```python
from build123d import *

# Parameters (mm, degrees)
BOX_W     = 13.4
BOX_H     = 13.4
BOX_DEPTH = 14


with BuildPart() as cube:
    # Box → Box (new body)
    with BuildSketch(Plane(origin=(-6.7, -6.7, 10), x_dir=(1, 0, 0), z_dir=(0, 0, 1))):
        with Locations((6.7, 6.7)):
            Rectangle(BOX_W, BOX_H)
    extrude(amount=BOX_DEPTH)


with BuildPart() as cut:
    # Sketch → Revolve (revolve)
    with BuildSketch(Plane.XZ):
        with BuildLine():
            Line((118.075, 18.37), (129.708369, 18.37))
            Line((129.708369, 18.37), (121.740684, 21.27))
            Line((121.740684, 21.27), (121.740684, 23.77))
            Line((121.740684, 23.77), (129.708369, 26.67))
            Line((129.708369, 26.67), (4.86, 26.67))
            Line((4.86, 26.67), (4.86, 10.010664))
            Line((4.86, 10.010664), (11.05, 10.010664))
            Line((11.05, 10.010664), (11.05, 18.37))
            add(Edge.make_bspline(
                [(118.075, 18.37), (77.146439, 24.763197), (51.362286, 25.0243), (11.05, 18.37)],
                knots=[0, 0, 0, 0, 1, 1, 1, 1], degree=3))
        make_face()
    revolve(axis=Axis((0, 0, 0), (0, 0, 1)))

    # Cut: cut Cube
    add(cube.part, mode=Mode.SUBTRACT)


solid = cut.part
```
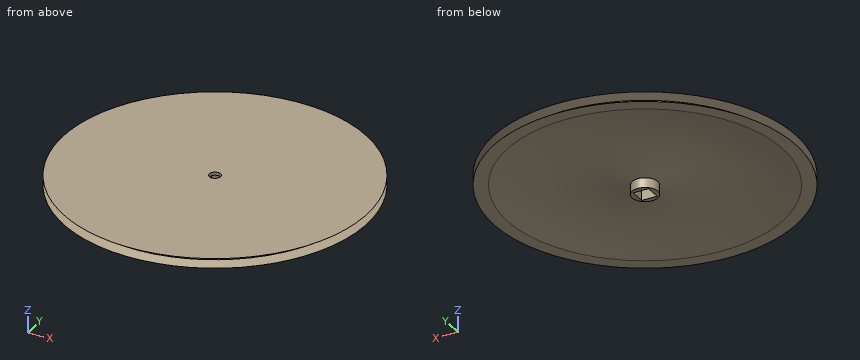
Geometry check sheet. Reference: the model listing, model coordinates, mm. Give positions to 0.01 mm unless a question says otherwise; leave off trailing zeros. Write each loop counter-clockwise with the first axis right and the second up, starting at its lowest first coordinate (ties: lowest second). Pieces come first, ordered by that corner, then holes.
1) Material ranges on L1, parallel to Z at x = -110, y = 29; L2, parallel to Z at x = 54, y = -58, recorded low to high.
2) Section check A-A, the plane z = 15.75. Record the boundary of the cut face in (x, y).
3) Gauge pin test, flat ends, axial feed: pin 1 (1 mm diameter, centred on x = -9, z = 15.5, fed in from +Y); pin 2 (4 mm diameter, centred on y = -1, z = 13.5, fed in from -X); pin 3 (10 mm diameter, centred on x = 10.5, y = -37.5, fed in from -Z). Record the tip position at first contact, or that the pin passes through.
Computed:
1. L1: z = 19.03 to 26.67
1. L2: z = 22.8 to 26.67
2. outline: circle Ø22.1 at (0, 0); hole (-6.7, -6.7) - (6.7, -6.7) - (6.7, 6.7) - (-6.7, 6.7) - close
3. pin 1: stops at y = 7.06
3. pin 2: stops at x = -11.05
3. pin 3: stops at z = 21.56
